from build123d import *

# Parameters (mm, degrees)
F1_DEPTH = 10
F2_D     = 4.2
F2_DEPTH = 7.4
F2_TIP   = 1.2618073


with BuildPart() as f1:
    # F0 (on Front) → F1 (new body)
    with BuildSketch(Plane.XZ):
        Polygon((35, -20), (35, 0), (35, 20), (-35, 20), (-35, -20), (-5.4585481157, -20), (-9.5, -27), (0, -27), (9.5, -27), (5.4585481157, -20), align=None)
    extrude(amount=F1_DEPTH)

    # F2
    with Locations(Plane(origin=(0, 0, 0), x_dir=(1, 0, 0), z_dir=(0, 1, 0))):
        with Locations((0, 0)):
            Hole(F2_D / 2, depth=F2_DEPTH)
            with Locations((0, 0, -(F2_DEPTH + F2_TIP / 2))):  # 118° drill point
                Cone(0, F2_D / 2, F2_TIP, mode=Mode.SUBTRACT)


solid = f1.part
Design review of the part built by this model. Coordinates are the model's own, in mm. A direction names the side the tool comes from. Give positions to 0.01 mm unless a question says otherwise; leave off trailing zeros. Order: outer loops, then holes, each group sorted by start corner. A loop starts at its lowest first (then second) coordinate and runs counter-clockwise, first axis right, second up.
1. Add section C-C, the plane x = 29. State the section outline as (y, z) points, then the cut area to 3 significant figures.
Solution:
outline: (-10, -20) - (0, -20) - (0, 20) - (-10, 20) - close
area: 400 mm2
2. Tool access review of faces 1 (the flat face through (-7.45, -4.93, -23.45)), 2 (the conical face through (0.35, -8.44, -0.11)): name each direction out of +Z, -Z, +X, -X, +Y, -Y from which nothing blocks a thin tool from reaching the whole face with its end or side.
Solution:
face 1: -X, +Y, -Y
face 2: +Y
3. Add section A-A, the plane y = -6.5. State the section outline as (x, z) points, then the cut area to 3 significant figures.
Solution:
outline: (-35, -20) - (-5.46, -20) - (-9.5, -27) - (9.5, -27) - (5.46, -20) - (35, -20) - (35, 20) - (-35, 20) - close; hole circle Ø4.2 at (0, 0)
area: 2,890 mm2
4. To check wall thickness, follow L1, parallel to Z at x = 0, y = -2; L2, parallel to Z at x = 19, y = -2; L3, parallel to Z at x = 7, y = -5. State the ranges of each line that lie inside material, in increasing order.
Solution:
L1: z = -27 to -2.1, 2.1 to 20
L2: z = -20 to 20
L3: z = -27 to -22.67, -20 to 20
5. Mouldability with a two-part tool opening along Z and no side actions: class faces 3 (the flat face through (0, -5, 20)), 4 (the cylindrical face through (-2.003, -3.752, -0.631)), 5 (the flat face through (0, -5, -27)), 6 (the flat face through (7.51, -4.93, -23.55)) as +Z half, -Z half, draft (parallel to the pull), parting line (faces both ways), or undercut.
Solution:
face 3: +Z half
face 4: undercut
face 5: -Z half
face 6: undercut
6. Add section D-D, the plane z = -23.5. State the section outline as (x, y) points.
Solution:
outline: (-7.48, -10) - (7.48, -10) - (7.48, 0) - (-7.48, 0) - close
7. For pin 1 Ø1 at (x, z) = (8.5, 13.5) entering from +Y; pin 2 Ø2 at (x, y) = (26, -8.5) entering from -Z; pin 3 Ø4 at (x, z) = (0, 0) entering from +Y, all flat-tipped, find the tip position at first contact; note any pin that passes through.
Solution:
pin 1: stops at y = 0
pin 2: stops at z = -20
pin 3: stops at y = -7.46
8. Add section B-B, the plane x = 7.5. State the section outline as (y, z) points.
Solution:
outline: (-10, -27) - (0, -27) - (0, -23.54) - (-10, -23.54) - close; (-10, -20) - (0, -20) - (0, 20) - (-10, 20) - close
